Check sheet for the modelled part. Datum: model origin and axes. Units: mm. Face numbers are marked on the shaded views. A direction names the side the tool comes from. Give positions to 0.01 mm unless a question says otherwise; leave off trailing zeros. Loops run counter-clockwise (first coordinate to the right, second up) from the corner with the lowest first, then second, coordinate; pieces in that order, holes last. Notation, with made-up numbers: (51, 77) -> (87, 77) arc R21 cw to (87, 86) -> close; hole circle Ø2 at (75.5, 24). An arc over 180 degrees is marked (long way). Write each question's results on one line, items separated by ' | '. Start each with the question number.
1. Material ranges on L1, parallel to Y at x = -29, z = 0; L2, parallel to X at y = 5, z = 4; L3, parallel to X at y = 26.5, z = 36, recorded low to high. Write a range as from..to.
2. Mould release check, pull along X, two halves, no side actions. Record for the marked faces 1, 2 and 3: +X half, -X half, draft (parallel to the pull), parting line (faces both ways), or undercut.
3. Tool access check on the marked faces 4, 5 and 6. Record the directions out of +Z, -Z, +X, -X, +Y, -Y that give a thin tool (end or side, any length) a straight path to the whole face; none if there is none.
4. Cross-section at C-C on y = 0. Record the boundary of the cut face in (x, z), and give its area (3 significant figures).
5. Gauge pin test, flat end, axial feed: pin 1 Ø8 at (x, z) = (4, -22.5) entering from +Y. Record the tip position at first contact, or that the pin passes through.
6. Cross-section at D-D on z = 20. Record the boundary of the cut face in (x, y).
7. Cross-section at B-B on z = -1. Record the boundary of the cut face in (x, y).
8. Cross-section at A-A on y = 20. Record the boundary of the cut face in (x, z), and give its area (3 significant figures).
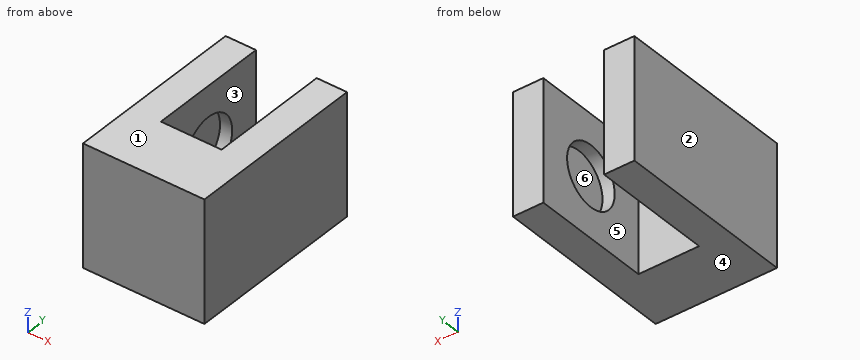
from build123d import *

# Parameters (mm, degrees)
EXTRUDE_1_DEPTH      = 50
EXTRUDE_1_DEPTH_BACK = 100
SKETCH_2_W           = 100
SKETCH_2_H           = 100
SKETCH_3_W           = 50
SKETCH_3_H           = 100
CUT_EXTRUDE_1_DEPTH  = 100
SKETCH_4_R           = 25
CUT_EXTRUDE_2_DEPTH  = 10
CUT_EXTRUDE_START    = -10
SKETCH_5_R           = 25
CUT_EXTRUDE_3_DEPTH  = 10


with BuildPart() as part:
    # 草图2 → 凸台-拉伸1 (new, two sides: drawn at the far end of the back side and taken through both)
    with BuildSketch(Plane(origin=(0, 0, 0), x_dir=(1, 0, 0), z_dir=(0, 1, 0)).offset(-EXTRUDE_1_DEPTH_BACK)):
        Rectangle(SKETCH_2_W, SKETCH_2_H)
    extrude(amount=EXTRUDE_1_DEPTH + EXTRUDE_1_DEPTH_BACK)

    # 草图3 → 切除-拉伸1 (cut)
    with BuildSketch(Plane(origin=(0, 50, 0), x_dir=(1, 0, 0), z_dir=(0, 1, 0))):
        Rectangle(SKETCH_3_W, SKETCH_3_H)
    extrude(amount=-CUT_EXTRUDE_1_DEPTH, mode=Mode.SUBTRACT)

    # 草图4 → 切除-拉伸2 (cut)
    with BuildSketch(Plane(origin=(-25, 0, 0), x_dir=(0, 0, -1), z_dir=(1, 0, 0))):
        Circle(SKETCH_4_R)
    extrude(amount=-CUT_EXTRUDE_2_DEPTH, mode=Mode.SUBTRACT)

    # 草图5 → 切除-拉伸3 (cut)
    with BuildSketch(Plane.ZY.offset(-25).offset(CUT_EXTRUDE_START)):
        with Locations(Location((0, 0, 0), (0, 0, 180))):
            Circle(SKETCH_5_R)
    extrude(amount=CUT_EXTRUDE_3_DEPTH, mode=Mode.SUBTRACT)


solid = part.part
Geometry says:
1) L1: -100..-25, 25..50 | L2: -50..-35, 35..50 | L3: -50..-25, 25..50
2) face 1: draft | face 2: -X half | face 3: undercut
3) face 4: -Z, +X, -X, +Y, -Y | face 5: +Z, -Z, +Y | face 6: none
4) outline: (-50, -50) -> (-25, -50) -> (-25, -25) -> (-35, -25) -> (-35, 25) -> (-25, 25) -> (-25, 50) -> (-50, 50) -> close; (25, -50) -> (50, -50) -> (50, 50) -> (25, 50) -> (25, 25) -> (35, 25) -> (35, -25) -> (25, -25) -> close | area: 4,000 mm^2
5) pin 1: y = -50
6) outline: (-50, -100) -> (50, -100) -> (50, 50) -> (25, 50) -> (25, 15) -> (35, 15) -> (35, -15) -> (25, -15) -> (25, -50) -> (-25, -50) -> (-25, -15) -> (-35, -15) -> (-35, 15) -> (-25, 15) -> (-25, 50) -> (-50, 50) -> close
7) outline: (-50, -100) -> (50, -100) -> (50, 50) -> (25, 50) -> (25, 24.98) -> (35, 24.98) -> (35, -24.98) -> (25, -24.98) -> (25, -50) -> (-25, -50) -> (-25, -24.98) -> (-35, -24.98) -> (-35, 24.98) -> (-25, 24.98) -> (-25, 50) -> (-50, 50) -> close
8) outline: (-50, -50) -> (-25, -50) -> (-25, -15) -> (-35, -15) -> (-35, 15) -> (-25, 15) -> (-25, 50) -> (-50, 50) -> close; (25, -50) -> (50, -50) -> (50, 50) -> (25, 50) -> (25, 15) -> (35, 15) -> (35, -15) -> (25, -15) -> close | area: 4,400 mm^2
